The model under review builds one solid part; all positions refer to its coordinate system, in mm. Face numbers are marked on the shaded views. Round coordinates to 2 decimals unless told otherwise and drop trailing zeros. Order: outer loops, then holes, each group sorted by start corner. A loop starts at its lowest first (then second) coordinate and runs counter-clockwise, first axis right, second up.
1) To check wall thickness, follow L1, parallel to Y at x = -206, z = 14 (3 decimals); L2, parallel to Y at x = -228.5, z = 6 (3 decimals); L3, parallel to Z at x = -195, y = 1.5. State the ranges of each line that lie inside material, in increasing order.
2) Clearance check with a flat-ended pin moving along its axis: P1, Ø1, axis at x = -205.5, y = -2.5, coming from the +Z side. State where the tip first meets the part, or that it passes through.
3) Consider section A-A (y = 66). Give the boundary of the cut face in (x, z).
4) Consider section C-C (z = 9.5). Give the number of separate pieces and of enclosed holes in the cut face, then the cut area to 3 significant figures.
5) Mouldability with a two-part tool opening along Y and no side actions: class the marked faces 1 and 2 as pulls with the +Y half, pulls with the -Y half, needs draft (parallel to the pull), parting line crosses it, or undercut.
6) Consider section D-D (y = -70). Give the boundary of the cut face in (x, z), then the cut area to 3 significant figures.
7) Consider section B-B (x = -50). Give the boundary of the cut face in (y, z) (3 decimals), then the cut area to 3 significant figures.
from build123d import *

# Parameters (mm, degrees)
SKETCH2_W           = 720
SKETCH2_H           = 279.33
BOSS_EXTRUDE1_DEPTH = 25
CUT_EXTRUDE1_DEPTH  = 22


with BuildPart() as part:
    # Sketch2 → Boss-Extrude1 (new body)
    with BuildSketch(Plane.XY):
        Rectangle(SKETCH2_W, SKETCH2_H)
    extrude(amount=BOSS_EXTRUDE1_DEPTH)

    # Sketch4 → Cut-Extrude1 (cut)
    with BuildSketch(Plane.XY.offset(25)):
        with BuildLine():
            Line((-326, 45), (-342.889989301, 45))
            ThreePointArc((-342.889989301, 45), (-344.341536559, 44.375867202), (-344.887125566, 42.893010557))
            Line((-344.887125566, 42.893010557), (-337.5, -95))
            Line((-337.5, -95), (-282.5, -95))
            Line((-282.5, -95), (-275.112874434, 42.893010557))
            ThreePointArc((-275.112874434, 42.893010557), (-275.658463441, 44.375867202), (-277.110010699, 45))
            Line((-277.110010699, 45), (-294, 45))
            Line((-294, 45), (-294, 95))
            Line((-294, 95), (-326, 95))
            Line((-326, 95), (-326, 45))
        make_face()
        with BuildLine():
            Line((-110.951497738, -95), (-103.564372172, 42.893010557))
            ThreePointArc((-103.564372172, 42.893010557), (-104.109961179, 44.375867202), (-105.561508437, 45))
            Line((-105.561508437, 45), (-122.451497738, 45))
            Line((-122.451497738, 45), (-122.451497738, 95))
            Line((-122.451497738, 95), (-154.451497738, 95))
            Line((-154.451497738, 95), (-154.451497738, 45))
            Line((-154.451497738, 45), (-171.341487039, 45))
            ThreePointArc((-171.341487039, 45), (-172.793034297, 44.375867202), (-173.338623303, 42.893010557))
            Line((-173.338623303, 42.893010557), (-165.951497738, -95))
            Line((-165.951497738, -95), (-110.951497738, -95))
        make_face()
        with BuildLine():
            Line((-259.112874434, 42.893010557), (-251.725748869, -95))
            Line((-251.725748869, -95), (-196.725748869, -95))
            Line((-196.725748869, -95), (-189.338623303, 42.893010557))
            ThreePointArc((-189.338623303, 42.893010557), (-189.88421231, 44.375867202), (-191.335759568, 45))
            Line((-191.335759568, 45), (-208.225748869, 45))
            Line((-208.225748869, 45), (-208.225748869, 95))
            Line((-208.225748869, 95), (-240.225748869, 95))
            Line((-240.225748869, 95), (-240.225748869, 45))
            Line((-240.225748869, 45), (-257.11573817, 45))
            ThreePointArc((-257.11573817, 45), (-258.567285428, 44.375867202), (-259.112874434, 42.893010557))
        make_face()
        with BuildLine():
            Line((-25.177246607, -95), (-17.790121041, 42.893010557))
            ThreePointArc((-17.790121041, 42.893010557), (-18.335710047, 44.375867202), (-19.787257306, 45))
            Line((-19.787257306, 45), (-36.677246607, 45))
            Line((-36.677246607, 45), (-36.677246607, 95))
            Line((-36.677246607, 95), (-68.677246607, 95))
            Line((-68.677246607, 95), (-68.677246607, 45))
            Line((-68.677246607, 45), (-85.567235908, 45))
            ThreePointArc((-85.567235908, 45), (-87.018783166, 44.375867202), (-87.564372172, 42.893010557))
            Line((-87.564372172, 42.893010557), (-80.177246607, -95))
            Line((-80.177246607, -95), (-25.177246607, -95))
        make_face()
        with BuildLine():
            Line((60.597004525, -95), (67.98413009, 42.893010557))
            ThreePointArc((67.98413009, 42.893010557), (67.438541084, 44.375867202), (65.986993826, 45))
            Line((65.986993826, 45), (49.097004525, 45))
            Line((49.097004525, 45), (49.097004525, 95))
            Line((49.097004525, 95), (17.097004525, 95))
            Line((17.097004525, 95), (17.097004525, 45))
            Line((17.097004525, 45), (0.207015224, 45))
            ThreePointArc((0.207015224, 45), (-1.244532035, 44.375867202), (-1.790121041, 42.893010557))
            Line((-1.790121041, 42.893010557), (5.597004525, -95))
            Line((5.597004525, -95), (60.597004525, -95))
        make_face()
        with BuildLine():
            Line((83.98413009, 42.893010557), (91.371255656, -95))
            Line((91.371255656, -95), (146.371255656, -95))
            Line((146.371255656, -95), (153.758381221, 42.893010557))
            ThreePointArc((153.758381221, 42.893010557), (153.212792215, 44.375867202), (151.761244957, 45))
            Line((151.761244957, 45), (134.871255656, 45))
            Line((134.871255656, 45), (134.871255656, 95))
            Line((134.871255656, 95), (102.871255656, 95))
            Line((102.871255656, 95), (102.871255656, 45))
            Line((102.871255656, 45), (85.981266355, 45))
            ThreePointArc((85.981266355, 45), (84.529719096, 44.375867202), (83.98413009, 42.893010557))
        make_face()
    extrude(amount=-CUT_EXTRUDE1_DEPTH, mode=Mode.SUBTRACT)


solid = part.part
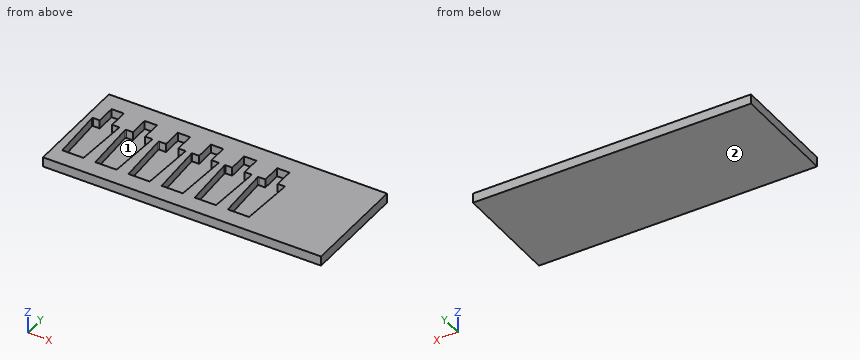
Answer below:
1. L1: y = -139.665 to -95, 45 to 139.665
1. L2: y = -139.665 to -95, 95 to 139.665
1. L3: z = 0 to 3
2. P1: stops at z = 3
3. outline: (-360, 0) - (360, 0) - (360, 25) - (134.87, 25) - (134.87, 3) - (102.87, 3) - (102.87, 25) - (49.1, 25) - (49.1, 3) - (17.1, 3) - (17.1, 25) - (-36.68, 25) - (-36.68, 3) - (-68.68, 3) - (-68.68, 25) - (-122.45, 25) - (-122.45, 3) - (-154.45, 3) - (-154.45, 25) - (-208.23, 25) - (-208.23, 3) - (-240.23, 3) - (-240.23, 25) - (-294, 25) - (-294, 3) - (-326, 3) - (-326, 25) - (-360, 25) - close
4. separate pieces: 1
4. enclosed holes: 6
4. area: 139,000 mm2
5. face 1: undercut
5. face 2: needs draft
6. outline: (-360, 0) - (360, 0) - (360, 25) - (147.71, 25) - (147.71, 3) - (90.03, 3) - (90.03, 25) - (61.94, 25) - (61.94, 3) - (4.26, 3) - (4.26, 25) - (-23.84, 25) - (-23.84, 3) - (-81.52, 3) - (-81.52, 25) - (-109.61, 25) - (-109.61, 3) - (-167.29, 3) - (-167.29, 25) - (-195.39, 25) - (-195.39, 3) - (-253.07, 3) - (-253.07, 25) - (-281.16, 25) - (-281.16, 3) - (-338.84, 3) - (-338.84, 25) - (-360, 25) - close
6. area: 10,400 mm2
7. outline: (-139.665, 0) - (139.665, 0) - (139.665, 25) - (95, 25) - (95, 3) - (-95, 3) - (-95, 25) - (-139.665, 25) - close
7. area: 2,800 mm2
